Design review of the part built by this model. Coordinates are the model's own, in mm. A direction names the side the tool comes from. Round coordinates to 2 decimals unless told otherwise and drop trailing zeros. Loops run counter-clockwise (first coordinate to the right, second up) from the corner with the lowest first, then second, coordinate; pieces in that order, holes last. Notation, with made-up numbers: M 19.25,78 L 26.25,78 A26 ccw 26.25,98 Z; hole C 38,39 d10. An arc over 180 degrees is marked long. Use a Markdown table: item, result.
from build123d import *

# Parameters (mm, degrees)
SKETCH1_R      = 4.0005
EXTRUDE1_DEPTH = 2.159
SKETCH2_R      = 2.032
EXTRUDE2_DEPTH = 8.89
EXTRUDE3_DEPTH = 1.016
CHAMFER1_SIZE  = 1.9558


with BuildPart() as part:
    # Sketch1 → Extrude1 (new body)
    with BuildSketch(Plane.XY):
        Circle(SKETCH1_R)
    extrude(amount=EXTRUDE1_DEPTH)

    # Sketch2 → Extrude2 (add)
    with BuildSketch(Plane.XY.offset(2.159)):
        Circle(SKETCH2_R)
    extrude(amount=EXTRUDE2_DEPTH)

    # Sketch3 → Extrude3 (cut)
    with BuildSketch(Plane(origin=(0, 0, 0), x_dir=(-1, 0, 0), z_dir=(0, 0, -1))):
        Polygon((1.206032038, 0.660002963), (0.031436687, 1.374455864), (-1.174595351, 0.714452901), (-1.206032038, -0.660002963), (-0.031436687, -1.374455864), (1.174595351, -0.714452901), align=None)
    extrude(amount=-EXTRUDE3_DEPTH, mode=Mode.SUBTRACT)

    # Chamfer1
    chamfer1_edges = [part.edges().sort_by_distance(p)[0] for p in [
        (-4.0005, 0, 2.159),
    ]]
    chamfer(chamfer1_edges, length=CHAMFER1_SIZE)


solid = part.part
1. Wall thickness on line 1 along Z through (x, y) = (1, 0); line 2 along X through (y, z) = (1.25, 0.5); line 3 along Z through (x, y) = (2.75, 2): over which ranges is each line inside the solid? List them lowest first. Write a range as from..to.
Check values:
| item | result |
|---|---|
| line 1 | z = 1.02..11.05 |
| line 2 | x = -3.49..-0.24, 0.2..3.49 |
| line 3 | z = 0..0.8 |
2. Insertion check: pin 1 (4 mm diameter, centred on y = 2, z = 3.5, fed in from +X); pin 2 (1 mm diameter, centred on x = 3, z = 8.5, fed in from -Y); pin 3 (0.7 mm diameter, centred on x = 0, y = 0.5, fed in from -Z). Each pin has a flat end and moves straight along its axis. Give the tip position at first contact, or say it passes through.
Check values:
| item | result |
|---|---|
| pin 1 | stops at x = 2.24 |
| pin 2 | passes through |
| pin 3 | stops at z = 1.02 |
3. Machinability: for faces 1 (the face through (0.63, -1.01, 0.5)), 2 (the face through (-0.44, -1.984, 6.542)), 3 (the face through (0, 0, 11.049)), which of the approach directions +Z, -Z, +X, -X, +Y, -Y give a long, thin tool a straight path to every point of the face, cutting with its end or side? Answer none if there is none.
Check values:
| item | result |
|---|---|
| face 1 | -Z |
| face 2 | +Z |
| face 3 | +Z, +X, -X, +Y, -Y |
4. Take a section at A-A on z = 7.5. Give the boundary of the cut face in (x, y).
Check values:
| item | result |
|---|---|
| outline | C 0,0 d4.06 |
